For this review, take the finished solid that the model builds, in its own axes (mm). A direction names the side the tool comes from. Coordinates: 2 decimals unless noted, no trailing zeros. Loops run counter-clockwise (first coordinate to the right, second up) from the corner with the lowest first, then second, coordinate; pieces in that order, holes last. Notation, with made-up numbers: M 43,27 L 47,27 A10 cw 47,42 Z; hole C -23,41.5 d7. An arc over 180 degrees is marked long. Use one line per item in the form item = value.
```python
from build123d import *

# Parameters (mm, degrees)
F1_DEPTH = 1
F0_W     = 120
F0_H     = 2
F2_DEPTH = 10
F3_D     = 4.5
F3_DEPTH = 2
F3_TIP   = 1.3519363928
F5_DEPTH = 13.5
F7_DEPTH = 13.5
F8_W     = 1
F8_H     = 10
F9_DEPTH = 2
F10_R    = 1


with BuildPart() as f1:
    # F0 (on Front) → F1 (new body)
    with BuildSketch(Plane.XZ):
        with BuildLine():
            Line((-60, 10), (-60, 0))
            Line((-60, 0), (60, 0))
            Line((60, 0), (60, 10))
            Line((60, 10), (55, 10))
            add(Edge.make_bspline(
                [(4.8726298846, 10), (8.1773018464, 3.085560631), (32.161216462, -1.0187632381), (50.9468838573, 3.4464653581), (55, 10)],
                knots=[0, 0, 0, 0, 0.5132056899, 1, 1, 1, 1], degree=3))
            Line((4.8726298846, 10), (-6.1437510885, 10))
            add(Edge.make_bspline(
                [(-55, 10), (-51.9492179155, 3.6175639834), (-34.2229071391, -1.2678204247), (-9.1991592199, 3.3849673346), (-6.1437510885, 10)],
                knots=[0, 0, 0, 0, 0.4730947214, 1, 1, 1, 1], degree=3))
            Line((-55, 10), (-60, 10))
        make_face()
    extrude(amount=-F1_DEPTH)

    # F0 (on Front) → F2 (join)
    with BuildSketch(Plane.XZ):
        with Locations((0, -1)):
            Rectangle(F0_W, F0_H)
    extrude(amount=-F2_DEPTH)

    # F3
    with Locations(Plane.XZ):
        with Locations((-55, 5), (-5, 5), (5, 5), (55, 5)):
            Hole(F3_D / 2, depth=F3_DEPTH)
            with Locations((0, 0, -(F3_DEPTH + F3_TIP / 2))):  # 118° drill point
                Cone(0, F3_D / 2, F3_TIP, mode=Mode.SUBTRACT)

    # F4 (on face) → F5 (join)
    with BuildSketch(Plane(origin=(-60, 0, 0), x_dir=(0, -1, 0), z_dir=(-1, 0, 0))):
        Polygon((-1, 0), (-10, 0), (-10, -2), (0, -2), (0, 0), align=None)
    extrude(amount=F5_DEPTH)

    # F6 (on face) → F7 (join)
    with BuildSketch(Plane.YZ.offset(60)):
        Polygon((0, 0), (0, -2), (10, -2), (10, 0), (1, 0), align=None)
    extrude(amount=F7_DEPTH)

    # F8 (on face) → F9 (join)
    with BuildSketch(Plane.XY):
        with Locations((-73, 5)):
            Rectangle(F8_W, F8_H)
        with Locations((73, 5)):
            Rectangle(F8_W, F8_H)
    extrude(amount=F9_DEPTH)

    # F10
    f10_edges = [f1.edges().sort_by_distance(p)[0] for p in [
        (0, 10, 0),
        (-66.25, 0, 0),
        (66.25, 0, 0),
    ]]
    fillet(f10_edges, radius=F10_R)


solid = f1.part
```
1. Tool access review of faces 1 (the face through (-1, 0, 1)), 2 (the face through (-1, 5, 0)): name each direction out of +Z, -Z, +X, -X, +Y, -Y from which nothing blocks a thin tool from reaching the whole face with its end or side.
Computed values:
face_1 = +Z, -Z, +X, -X, -Y
face_2 = +Z, +Y
2. For pin 1 Ø3 at (x, y) = (5.5, 4.5) entering from +Z; pin 2 Ø6 at (y, z) = (1, 6.5) entering from -X; pin 3 Ø2 at (x, z) = (13.5, 3) entering from -Y; pin 4 Ø5 at (x, z) = (5, 5) entering from +Y, all flat-tipped, find the tip position at first contact; note any pin that passes through.
Computed values:
pin_1 = 0
pin_2 = -60
pin_3 = 0
pin_4 = 1
3. Consider section C-C on z = 5. State how many separate pieces and enclosed holes the cut face has, plus the area to 3 significant figures.
Computed values:
separate_pieces = 7
enclosed_holes = 0
area = 23.4 mm2
4. Consider section B-B on x = 62. Write out the cut boundary in (y, z), plus the area to 3 significant figures.
Computed values:
outline = M 0,-2 L 10,-2 L 10,-1 A1 ccw 9,0 L 1,0 A1 ccw 0,-1 Z
area = 19.6 mm2
5. Consider section A-A on y = 4.5. Write out the cut boundary in (x, z).
Computed values:
outline = M -73.5,-2 L 73.5,-2 L 73.5,2 L 72.5,2 L 72.5,0 L -72.5,0 L -72.5,2 L -73.5,2 Z
6. Wall thickness on line 1 along Z through (x, y) = (-5, 0.2); line 2 along X through (y, z) = (2.75, 0.25); line 3 along Z through (x, y) = (41.5, 6.25): over which ranges is each line inside the solid? List them lowest first. Write a range as from..to.
Computed values:
line_1 = -2..2.75, 7.25..10
line_2 = -73.5..-72.5, 72.5..73.5
line_3 = -2..0
7. Draft analysis for pull direction X (two halves, no side actions). For faces 3 (the face through (-1, 5, -2)), 4 (the face through (73.5, 5, 0)), 5 (the face through (-52.752, 0.507, 5.099)), state which applies: +X half, -X half, draft (parallel to the pull), parting line (faces both ways), or undercut.
Computed values:
face_3 = draft
face_4 = +X half
face_5 = undercut
